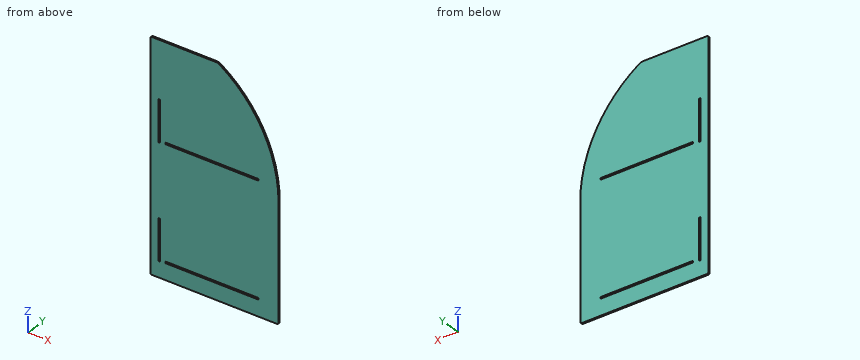
from build123d import *

# Parameters (mm, degrees)
F0_W     = 5
F0_H     = 127
F0_W_2   = 289
F0_H_2   = 5
F1_DEPTH = 5


with BuildPart() as f1:
    # F0 (on Front) → F1 (new body)
    with BuildSketch(Plane.XZ):
        with BuildLine():
            ThreePointArc((0, 5), (1.464466, 1.464466), (5, 0))
            Line((5, 0), (395, 0))
            ThreePointArc((395, 0), (398.535534, 1.464466), (400, 5))
            Line((400, 5), (400, 360))
            ThreePointArc((400, 360), (350.920298, 551.976416), (215.725279, 696.842105))
            ThreePointArc((215.725279, 696.842105), (210.55853, 699.194297), (204.939015, 700))
            Line((204.939015, 700), (5, 700))
            ThreePointArc((5, 700), (1.464466, 698.535534), (0, 695))
            Line((0, 695), (0, 5))
        make_face()
        with Locations((27.5, 111.5)):
            Rectangle(F0_W, F0_H, mode=Mode.SUBTRACT)
        with Locations((192.5, 52.5)):
            Rectangle(F0_W_2, F0_H_2, mode=Mode.SUBTRACT)
        with Locations((27.5, 461.5)):
            Rectangle(F0_W, F0_H, mode=Mode.SUBTRACT)
        with Locations((192.5, 402.5)):
            Rectangle(F0_W_2, F0_H_2, mode=Mode.SUBTRACT)
    extrude(amount=F1_DEPTH)


solid = f1.part
Work out the finished part from the listing and answer in its coordinate system (mm). Give positions to 0.01 mm unless a question says otherwise; leave off trailing zeros. Loops run counter-clockwise (first coordinate to the right, second up) from the corner with the lowest first, then second, coordinate; pieces in that order, holes last. Notation, with made-up numbers: (45.25, -33) -> (64.25, -33) arc R32 cw to (64.25, 3) -> close; hole circle Ø8 at (50.5, 48.5). An arc over 180 degrees is marked (long way). Use a Markdown table: item, result. Add a question column.
1. Section A-A on z = 512 is taken. Determine the outline of the cut face in (x, y), and give its area (3 significant figures).
2. Section C-C on x = 241 is taken. Determine the outline of the cut face in (y, z), and give its area (3 significant figures).
3. A flat-ended cylindrical pin translates along its axis: pin 1 Ø1.5 at (y, z) = (-3.5, 438.5) entering from +X. Find the tip coordinate at first contact, or state that the pin passes through.
4. Find the intervals of material crossed by probe 1 along Z at (x, y) = (197, -3.4); probe 2 along Z at (x, y) = (220.5, -2.2); probe 3 along X at (y, z) = (-4.3, 78), in increasing order.
5. Section B-B on y = -1.7 is taken. Determine the outline of the cut face in (x, z), and give its area (3 significant figures).
6. Section D-D on x = 292 is taken. Determine the outline of the cut face in (y, z), and give its area (3 significant figures).
Results below:
| question | item | result |
|---|---|---|
| 1 | outline | (0, -5) -> (25, -5) -> (25, 0) -> (0, 0) -> close; (30, -5) -> (369.99, -5) -> (369.99, 0) -> (30, 0) -> close |
| 1 | area | 1,820 mm^2 |
| 2 | outline | (-5, 0) -> (0, 0) -> (0, 50) -> (-5, 50) -> close; (-5, 55) -> (0, 55) -> (0, 400) -> (-5, 400) -> close; (-5, 405) -> (0, 405) -> (0, 679.25) -> (-5, 679.25) -> close |
| 2 | area | 3,350 mm^2 |
| 3 | pin 1 | stops at x = 392.37 |
| 4 | probe 1 | z = 0 to 50, 55 to 400, 405 to 700 |
| 4 | probe 2 | z = 0 to 50, 55 to 400, 405 to 693.74 |
| 4 | probe 3 | x = 0 to 25, 30 to 400 |
| 5 | outline | (0, 5) arc R5 ccw to (5, 0) -> (395, 0) arc R5 ccw to (400, 5) -> (400, 360) arc R400 ccw to (215.73, 696.84) arc R20 ccw to (204.94, 700) -> (5, 700) arc R5 ccw to (0, 695) -> close; hole (25, 48) -> (30, 48) -> (30, 175) -> (25, 175) -> close; hole (25, 398) -> (30, 398) -> (30, 525) -> (25, 525) -> close; hole (48, 50) -> (337, 50) -> (337, 55) -> (48, 55) -> close; hole (48, 400) -> (337, 400) -> (337, 405) -> (48, 405) -> close |
| 5 | area | 257,000 mm^2 |
| 6 | outline | (-5, 0) -> (0, 0) -> (0, 50) -> (-5, 50) -> close; (-5, 55) -> (0, 55) -> (0, 400) -> (-5, 400) -> close; (-5, 405) -> (0, 405) -> (0, 633.38) -> (-5, 633.38) -> close |
| 6 | area | 3,120 mm^2 |
